For this review, take the finished solid that the model builds, in its own axes (mm). Face numbers are marked on the shaded views. Give positions to 0.01 mm unless a question says otherwise; leave off trailing zeros. Order: outer loops, then holes, each group sorted by start corner. A loop starts at its lowest first (then second) coordinate and runs counter-clockwise, first axis right, second up.
Item 1: The part is to be moulded in two halves that separate along Z. For the marked faces 1, 2 and 3, say which applies: released by +Z, released by -Z, zero draft, split by the parting line, or undercut.
Item 2: For P1, Ø2.5, axis at x = 1.5, y = 7.5, coming from the +Z side; P2, Ø1.9, axis at y = 4, z = -4.5, coming from the +X side; P3, Ø10, axis at x = 10, z = 2.5, coming from the +Y side, all flat-tipped, find the tip position at first contact; note any pin that passes through.
Item 3: For probe 1 along X at (y, z) = (4.75, 0); probe 2 along Y at (x, z) = (9.25, -4.75); probe 3 along X at (y, z) = (5.75, -11.75), list the stretches that pass through material, from the lowest coordinate up.
Item 4: Consider section B-B (y = 5.5). Give the boundary of the cut face in (x, z), plus the area to 3 significant figures.
Item 5: Consider section A-A (y = 13). Give the boundary of the cut face in (x, z), plus the area to 3 significant figures.
Item 6: Consider section D-D (x = 5). Give the boundary of the cut face in (y, z).
```python
from build123d import *

# Parameters (mm, degrees)
SKETCH_1_R      = 15
EXTRUDE_1_DEPTH = 8.6
SHELL_1_T       = -1.6
SKETCH_2_R      = 6.75
SKETCH_2_R_2    = 5.75
EXTRUDE_2_DEPTH = 8.8
EXTRUDE_4_DEPTH = 3.6
EXTRUDE_7_DEPTH = 1.5
FILLET_2_R      = 1.5
EXTRUDE_8_DEPTH = 9.7


with BuildPart() as part:
    # 草图1 → 凸台-拉伸1 (new body)
    with BuildSketch(Plane(origin=(0, 0, 0), x_dir=(1, 0, 0), z_dir=(0, 1, 0))):
        with Locations(Location((0, 0, 0), (0, 0, 90))):
            Circle(SKETCH_1_R)
    extrude(amount=EXTRUDE_1_DEPTH)

    # 抽壳1
    shell_1_openings = [part.faces().sort_by_distance(p)[0] for p in [
        (0, 8.6, 0),
    ]]
    offset(amount=SHELL_1_T, openings=shell_1_openings, kind=Kind.INTERSECTION)

    # 草图2 → 凸台-拉伸2 (add)
    with BuildSketch(Plane(origin=(0, 1.6, 0), x_dir=(1, 0, 0), z_dir=(0, 1, 0))):
        with Locations(Location((0, 0, 0), (0, 0, 270))):
            Circle(SKETCH_2_R)
        with Locations(Location((0, 0, 0), (0, 0, 270))):
            Circle(SKETCH_2_R_2, mode=Mode.SUBTRACT)
    extrude(amount=EXTRUDE_2_DEPTH)

    # 草图5 → 凸台-拉伸4 (add)
    with BuildSketch(Plane(origin=(0, 10.4, 0), x_dir=(1, 0, 0), z_dir=(0, 1, 0))):
        with BuildLine():
            Line((-6.229165273, 2.6), (-5.407902558, 1.954279393))
            ThreePointArc((-5.407902558, 1.954279393), (-5.750152822, 0.018988088), (-5.420691276, -1.918521336))
            Line((-5.420691276, -1.918521336), (-6.224112, -2.612073854))
            ThreePointArc((-6.224112, -2.612073854), (-6.749996828, -0.006544339), (-6.229165273, 2.6))
        make_face()
        with BuildLine():
            Line((-3.75, 5.61248608), (-2.937259379, 4.943392091))
            ThreePointArc((-2.937259379, 4.943392091), (0, 5.750184173), (2.937259379, 4.943392091))
            Line((2.937259379, 4.943392091), (3.75, 5.61248608))
            ThreePointArc((3.75, 5.61248608), (0, 6.75), (-3.75, 5.61248608))
        make_face()
        with BuildLine():
            Line((6.229165273, 2.6), (5.416190763, 1.931190215))
            ThreePointArc((5.416190763, 1.931190215), (5.750184173, 0), (5.416190763, -1.931190215))
            Line((5.416190763, -1.931190215), (6.229165273, -2.6))
            ThreePointArc((6.229165273, -2.6), (6.75, 0), (6.229165273, 2.6))
        make_face()
        with BuildLine():
            Line((3.75, -5.61248608), (2.937259379, -4.943392091))
            ThreePointArc((2.937259379, -4.943392091), (0, -5.750184173), (-2.937259379, -4.943392091))
            Line((-2.937259379, -4.943392091), (-3.75, -5.61248608))
            ThreePointArc((-3.75, -5.61248608), (0, -6.75), (3.75, -5.61248608))
        make_face()
    extrude(amount=EXTRUDE_4_DEPTH)

    # 草图14 → 凸台-拉伸7 (add)
    with BuildSketch(Plane(origin=(0, 14, 0), x_dir=(1, 0, 0), z_dir=(0, 1, 0))):
        with BuildLine():
            Line((-4.551719875, 6.272507169), (-3.75, 5.61248608))
            Line((-3.75, 5.61248608), (-2.937108239, 4.943267664))
            ThreePointArc((-2.937108239, 4.943267664), (-0.000121801, 5.749999999), (2.936898812, 4.943392091))
            Line((2.936898812, 4.943392091), (3.75, 5.61248608))
            Line((3.75, 5.61248608), (4.551908877, 6.272370013))
            ThreePointArc((4.551908877, 6.272370013), (0.000116762, 7.749999999), (-4.551719875, 6.272507169))
        make_face()
        with BuildLine():
            Line((4.551908877, -6.272370013), (3.75, -5.61248608))
            Line((3.75, -5.61248608), (2.936898812, -4.943392091))
            ThreePointArc((2.936898812, -4.943392091), (-0.000121801, -5.749999999), (-2.937108239, -4.943267664))
            Line((-2.937108239, -4.943267664), (-3.75, -5.61248608))
            Line((-3.75, -5.61248608), (-4.551719875, -6.272507169))
            ThreePointArc((-4.551719875, -6.272507169), (0.000116762, -7.749999999), (4.551908877, -6.272370013))
        make_face()
    extrude(amount=EXTRUDE_7_DEPTH)

    # 圆角2
    fillet_2_edges = [part.edges().sort_by_distance(p)[0] for p in [
        (0.000116762, 15.5, 7.749999999),
        (0.000116762, 15.5, -7.749999999),
    ]]
    fillet(fillet_2_edges, radius=FILLET_2_R - 0.0001)  # a hair under: the kernel refuses the full size

    # 草图15 → 凸台-拉伸8 (add)
    with BuildSketch(Plane(origin=(0, 1.6, 0), x_dir=(1, 0, 0), z_dir=(0, 1, 0))):
        with BuildLine():
            Line((-2.645751311, -3), (-0.4, -3))
            Line((-0.4, -3), (-0.4, -5.736070083))
            ThreePointArc((-0.4, -5.736070083), (0, -5.75), (0.4, -5.736070083))
            Line((0.4, -5.736070083), (0.4, -3))
            Line((0.4, -3), (2.645751311, -3))
            ThreePointArc((2.645751311, -3), (3.807765077, 1.22512249), (0.4, 3.979949748))
            Line((0.4, 3.979949748), (0.4, 5.736070083))
            ThreePointArc((0.4, 5.736070083), (0, 5.75), (-0.4, 5.736070083))
            Line((-0.4, 5.736070083), (-0.4, 3.979949748))
            ThreePointArc((-0.4, 3.979949748), (-3.807765077, 1.22512249), (-2.645751311, -3))
        make_face()
        with BuildLine():
            Line((1.407515289, -2), (0.4, -2))
            Line((0.4, -2), (-0.4, -2))
            Line((-0.4, -2), (-2.236067977, -2))
            ThreePointArc((-2.236067977, -2), (0, 3), (2.236067977, -2))
            Line((2.236067977, -2), (1.407515289, -2))
        make_face(mode=Mode.SUBTRACT)
    extrude(amount=EXTRUDE_8_DEPTH)


solid = part.part
```
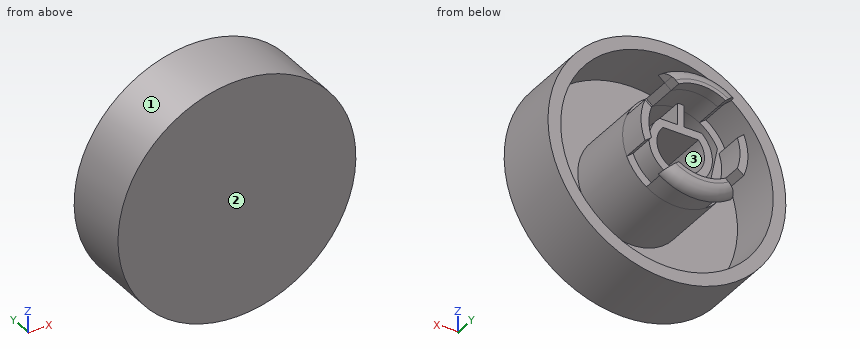
Resolved:
1. face 1: split by the parting line
1. face 2: zero draft
1. face 3: undercut
2. P1: stops at z = 15
2. P2: stops at x = 14.57
2. P3: stops at y = 14
3. probe 1: x = -15 to -13.4, -6.75 to -5.75, -4 to -3, 3 to 4, 5.75 to 6.75, 13.4 to 15
3. probe 2: y = 0 to 1.6
3. probe 3: x = -9.32 to -6.44, 6.44 to 9.32
4. outline: circle Ø30 at (0, 0); circle Ø13.5 at (0, 0); hole circle Ø26.8 at (0, 0); hole (-2.65, 3) - (-0.4, 3) - (-0.4, 5.74) arc R5.75 ccw to (-0.4, -5.74) - (-0.4, -3.98) arc R4 cw to start; hole (-2.24, 2) arc R3 ccw (long way) to (2.24, 2) - close; hole (0.4, -5.74) arc R5.75 ccw to (0.4, 5.74) - (0.4, 3) - (2.65, 3) arc R4 cw to (0.4, -3.98) - close
4. area: 207 mm2
5. outline: (-6.23, -2.6) - (-5.41, -1.95) arc R5.75 cw to (-5.42, 1.92) - (-6.22, 2.61) arc R6.75 ccw to start; (-3.75, -5.61) arc R6.75 ccw to (3.75, -5.61) - (2.94, -4.94) arc R5.75 cw to (-2.94, -4.94) - close; (-3.75, 5.61) - (-2.94, 4.94) arc R5.75 cw to (2.94, 4.94) - (3.75, 5.61) arc R6.75 ccw to start; (5.42, -1.93) - (6.23, -2.6) arc R6.75 ccw to (6.23, 2.6) - (5.42, 1.93) arc R5.75 cw to start
5. area: 23.4 mm2
6. outline: (0, -14.14) - (8.6, -14.14) - (8.6, -12.43) - (1.6, -12.43) - (1.6, -4.53) - (10.4, -4.53) - (10.4, -2.84) - (1.6, -2.84) - (1.6, 2.84) - (10.4, 2.84) - (10.4, 4.53) - (1.6, 4.53) - (1.6, 12.43) - (8.6, 12.43) - (8.6, 14.14) - (0, 14.14) - close
